Geometry: final body of the model. Coordinates: model frame, mm. A direction names the side the tool comes from. Coordinates: 2 decimals unless noted, no trailing zeros. Order: outer loops, then holes, each group sorted by start corner. A loop starts at its lowest first (then second) coordinate and runs counter-clockwise, first axis right, second up. Notation, with made-up numbers: (2, 15) -> (55, 15) arc R20 ccw to (55, 29) -> close; hole circle Ø10 at (22, 78). An arc over 180 degrees is marked (long way). Use one line per item in the form item = value.
```python
from build123d import *

# Parameters (mm, degrees)
SKETCH1_W           = 170
SKETCH1_H           = 58
BOSS_EXTRUDE1_DEPTH = 5
SKETCH2_W           = 28
SKETCH2_H           = 58
BOSS_EXTRUDE2_DEPTH = 25
CUT_EXTRUDE4_DEPTH  = 25
HOLE1_START         = -29
HOLE1_OUTLINE_R     = 5
HOLE1_DEPTH         = 58
SKETCH6_W           = 16
SKETCH6_H           = 58
BOSS_EXTRUDE3_DEPTH = 60
SKETCH7_W           = 1.2
SKETCH7_H           = 58
CUT_EXTRUDE5_DEPTH  = 62
SKETCH8_R           = 5.5
CUT_EXTRUDE6_DEPTH  = 100
SKETCH9_R           = 1.8
CUT_EXTRUDE7_DEPTH  = 20
HOLE3_START         = -20
HOLE3_OUTLINE_R     = 5
HOLE3_DEPTH         = 39.8


# Read off the part's stored shape, not the designer's step: Hole1, Hole3
with BuildPart() as part:
    # Sketch1 → Boss-Extrude1 (new body)
    with BuildSketch(Plane.XY):
        Rectangle(SKETCH1_W, SKETCH1_H)
    extrude(amount=BOSS_EXTRUDE1_DEPTH)

    # Sketch2 → Boss-Extrude2 (add)
    with BuildSketch(Plane(origin=(0, 0, 5), x_dir=(-1, 0, 0), z_dir=(0, 0, -1))):
        with Locations((71, 0)):
            Rectangle(SKETCH2_W, SKETCH2_H)
        with Locations((-71, 0)):
            Rectangle(SKETCH2_W, SKETCH2_H)
    extrude(amount=-BOSS_EXTRUDE2_DEPTH)

    # Sketch3 → Cut-Extrude4 (cut)
    with BuildSketch(Plane.XY.offset(30)):
        Polygon((-57, -29), (-57, -20), (-77, -20), (-76.8, 19.8), (-57, 19.8), (-57, 29), (-85, 29), (-85, -29), align=None)
        Polygon((56, 8.9), (56, 18.1), (76.8, 18.1), (76.8, 29), (85, 29), (85, -29), (76.8, -29), (76.8, -18.1), (56, -18.1), (56, -8.9), (76.8, -8.9), (76.8, 8.9), align=None)
    extrude(amount=-CUT_EXTRUDE4_DEPTH, mode=Mode.SUBTRACT)

    # Hole1 outline → Hole1 (cut)
    with BuildSketch(Plane(origin=(0, 0, 0), x_dir=(1, 0, 0), z_dir=(0, 1, 0)).offset(HOLE1_START)):
        with Locations((67.918134457, -16.770132162)):
            Circle(HOLE1_OUTLINE_R)
    extrude(amount=HOLE1_DEPTH, mode=Mode.SUBTRACT)

    # Sketch6 → Boss-Extrude3 (add)
    with BuildSketch(Plane.XY.offset(5)):
        with Locations((-10, 0)):
            Rectangle(SKETCH6_W, SKETCH6_H)
    extrude(amount=BOSS_EXTRUDE3_DEPTH)

    # Sketch7 → Cut-Extrude5 (cut)
    with BuildSketch(Plane(origin=(0, 0, 0), x_dir=(-1, 0, 0), z_dir=(0, 0, -1))):
        with Locations((10, 0)):
            Rectangle(SKETCH7_W, SKETCH7_H)
    extrude(amount=-CUT_EXTRUDE5_DEPTH, mode=Mode.SUBTRACT)

    # Sketch8 → Cut-Extrude6 (cut)
    with BuildSketch(Plane(origin=(0, 0, 0), x_dir=(-1, 0, 0), z_dir=(0, 0, -1))):
        with Locations(Location((10, 0, 0), (0, 0, 83.737086874))):
            Circle(SKETCH8_R)
    extrude(amount=-CUT_EXTRUDE6_DEPTH, mode=Mode.SUBTRACT)

    # Sketch9 → Cut-Extrude7 (cut)
    with BuildSketch(Plane.ZY.offset(18)):
        with Locations((34, 12)):
            Circle(SKETCH9_R)
        with Locations((10, 12)):
            Circle(SKETCH9_R)
        with Locations((10, -12)):
            Circle(SKETCH9_R)
        with Locations((34, -12)):
            Circle(SKETCH9_R)
    extrude(amount=-CUT_EXTRUDE7_DEPTH, mode=Mode.SUBTRACT)

    # Hole3 outline → Hole3 (cut)
    with BuildSketch(Plane(origin=(0, 0, 0), x_dir=(1, 0, 0), z_dir=(0, 1, 0)).offset(HOLE3_START)):
        with Locations((-68.081865543, -16.770132162)):
            Circle(HOLE3_OUTLINE_R)
    extrude(amount=HOLE3_DEPTH, mode=Mode.SUBTRACT)


solid = part.part
```
1) Section C-C, the plane z = 43.5. Output: boundary loops of the cut face in (x, y).
Results found:
outline = (-18, -29) -> (-10.6, -29) -> (-10.6, -5.47) arc R5.5 cw to (-10.6, 5.47) -> (-10.6, 29) -> (-18, 29) -> close; (-9.4, -29) -> (-2, -29) -> (-2, 29) -> (-9.4, 29) -> (-9.4, 5.47) arc R5.5 cw to (-9.4, -5.47) -> close
2) Pull-direction query (X, two-part tool) for faces 1 (the flat face through (-48, 0, 0)), 2 (the cylindrical face through (-15.207, -1.771, 32.045)); classes: released by +X, released by -X, zero draft, split by the parting line, or undercut.
Results found:
face_1 = zero draft
face_2 = undercut
3) Section B-B, the plane y = 0. Output: boundary loops of the cut face in (x, z).
Results found:
outline = (-85, 0) -> (-15.5, 0) -> (-15.5, 65) -> (-18, 65) -> (-18, 5) -> (-57, 5) -> (-57, 30) -> (-76.9, 30) -> (-76.9, 5) -> (-85, 5) -> close; (-4.5, 0) -> (85, 0) -> (85, 5) -> (76.8, 5) -> (76.8, 30) -> (57, 30) -> (57, 5) -> (-2, 5) -> (-2, 65) -> (-4.5, 65) -> close; hole circle Ø10 at (-68.08, 16.77); hole circle Ø10 at (67.92, 16.77)
4) Contact query for flat-ended pins moving along their axis: P1, Ø1.5, axis at y = 7, z = 40.5, coming from the +X side; P2, Ø19, axis at y = 19, z = 20.5, coming from the +X side; P3, Ø14, axis at x = 63, y = -1.5, coming from the +Z side. Output: stop coordinate, or through.
Results found:
P1 = -2
P2 = 76.8
P3 = 30
5) Section A-A, the plane z = 34. Output: boundary loops of the cut face in (x, y).
Results found:
outline = (-18, -29) -> (-10.6, -29) -> (-10.6, -13.8) -> (-18, -13.8) -> close; (-18, -10.2) -> (-10.6, -10.2) -> (-10.6, -5.47) arc R5.5 cw to (-10.6, 5.47) -> (-10.6, 10.2) -> (-18, 10.2) -> close; (-18, 13.8) -> (-10.6, 13.8) -> (-10.6, 29) -> (-18, 29) -> close; (-9.4, -29) -> (-2, -29) -> (-2, -13.8) -> (-9.4, -13.8) -> close; (-9.4, -10.2) -> (-2, -10.2) -> (-2, 10.2) -> (-9.4, 10.2) -> (-9.4, 5.47) arc R5.5 cw to (-9.4, -5.47) -> close; (-9.4, 13.8) -> (-2, 13.8) -> (-2, 29) -> (-9.4, 29) -> close
6) Section D-D, the plane z = 10. Give the number of separate pieces and of enclosed holes in the cut face, and give its area (3 significant figures).
Results found:
separate_pieces = 10
enclosed_holes = 0
area = 2,250 mm2
7) Material intervals for probe 1 along Y at (x, z) = (-4, 34); probe 2 along X at (y, z) = (20, 31); probe 3 along X at (y, z) = (-25.5, 4.5), sorted ascending. Write a range as from..to.
Results found:
probe_1 = -29..-13.8, -10.2..10.2, 13.8..29
probe_2 = -18..-10.6, -9.4..-2
probe_3 = -85..-10.6, -9.4..85
8) Access query for faces 3 (the flat face through (-2, 0, 35)), 4 (the flat face through (-9.4, -17, 31)), 5 (the cylindrical face through (-5.75, 12.08, 8.2)), 6 (the flat face through (62.6, 8.9, 17.7)). Directions: +Z, -Z, +X, -X, +Y, -Y. A direction counts if a zero-diameter tool reaches every point of the face in a straight line with its end or side. Return the directions, or none.
Results found:
face_3 = +Z, +Y, -Y
face_4 = -Z, +Y, -Y
face_5 = +X
face_6 = +Z, +X
